Source: CAD feature listing. Evaluate the final solid. Frame: model axes, mm. A direction names the side the tool comes from. Give positions to 0.01 mm unless a question says otherwise; leave off trailing zeros. Order: outer loops, then holes, each group sorted by start corner. A loop starts at its lowest first (then second) coordinate and runs counter-clockwise, first axis right, second up.
Autodesk Inventor part; units mm, degrees
ref_plane "bolt4_1_XY" through (-10, 3.5, 10) normal (0, 1, 0) x (1, 0, 0)
ref_plane "bolt4_1_YZ" through (-10, 3.5, 10) normal (1, 0, 0) x (0, 0, -1)
ref_plane "bolt4_1_ZX" through (-10, 3.5, 10) normal (0, 0, -1) x (0, 1, 0)
sketch "Sketch_4" plane through (0, 0, 0) normal (0, 1, 0) x (-1, 0, 0)
  line L0 (40, -19) -> (40, 19)
  line L1 (40, 19) -> (39, 20)
  line L2 (39, 20) -> (-39, 20)
  line L3 (-39, 20) -> (-40, 19)
  line L4 (-40, 19) -> (-40, -19)
  line L5 (-40, -19) -> (-39, -20)
  line L6 (-39, -20) -> (39, -20)
  line L7 (39, -20) -> (40, -19)
extrude "Extrusion1" add sketch "Sketch_4" along normal blind 9
sketch "Sketch2" plane through (0, 0, 0) normal (0, -1, 0) x (1, 0, 0)
  point P0 (-30, 10)
hole "Hole1" at (-30, 0, 10) direction (0, 1, 0) diameter 5.5 depth 9 counterbore diameter 9.5 counterbore depth 5.5
pattern_linear "Rectangular Pattern1" count 2 spacing 60 along (1, 0, 0) count 2 spacing 20 along (0, 0, -1) of "Hole1"
sketch "Sketch3" plane through (0, 9, 0) normal (0, 1, 0) x (1, 0, 0)
  point P0 (-10, -10)
hole "Hole2" at (-10, 9, 10) direction (0, -1, 0) diameter 5.5 depth 9 counterbore diameter 9.5 counterbore depth 5.5
pattern_linear "Rectangular Pattern2" count 2 spacing 20 along (1, 0, 0) count 2 spacing 20 along (0, 0, -1) of "Hole2"
ref_plane "bolt4_1_XY" through (-10, 3.5, 10) normal (0, 1, 0) x (1, 0, 0)
ref_plane "bolt4_1_YZ" through (-10, 3.5, 10) normal (1, 0, 0) x (0, 0, -1)
ref_plane "bolt4_1_ZX" through (-10, 3.5, 10) normal (0, 0, -1) x (0, 1, 0)
ref_plane "bolt4_2_XY" through (10, 3.5, 10) normal (0, 1, 0) x (1, 0, 0)
ref_plane "bolt4_2_YZ" through (10, 3.5, 10) normal (1, 0, 0) x (0, 0, -1)
ref_plane "bolt4_2_ZX" through (10, 3.5, 10) normal (0, 0, -1) x (0, 1, 0)
ref_plane "bolt4_3_XY" through (-10, 3.5, -10) normal (0, 1, 0) x (1, 0, 0)
ref_plane "bolt4_3_YZ" through (-10, 3.5, -10) normal (1, 0, 0) x (0, 0, -1)
ref_plane "bolt4_3_ZX" through (-10, 3.5, -10) normal (0, 0, -1) x (0, 1, 0)
ref_plane "bolt4_4_XY" through (10, 3.5, -10) normal (0, 1, 0) x (1, 0, 0)
ref_plane "bolt4_4_YZ" through (10, 3.5, -10) normal (1, 0, 0) x (0, 0, -1)
ref_plane "bolt4_4_ZX" through (10, 3.5, -10) normal (0, 0, -1) x (0, 1, 0)
ref_plane "bolt5_1_XY" through (-30, 5.5, 10) normal (0, 1, 0) x (1, 0, 0)
ref_plane "bolt5_1_YZ" through (-30, 5.5, 10) normal (1, 0, 0) x (0, 0, -1)
ref_plane "bolt5_1_ZX" through (-30, 5.5, 10) normal (0, 0, -1) x (0, 1, 0)
ref_plane "bolt5_2_XY" through (30, 5.5, 10) normal (0, 1, 0) x (1, 0, 0)
ref_plane "bolt5_2_YZ" through (30, 5.5, 10) normal (1, 0, 0) x (0, 0, -1)
ref_plane "bolt5_2_ZX" through (30, 5.5, 10) normal (0, 0, -1) x (0, 1, 0)
ref_plane "bolt5_3_XY" through (-30, 5.5, -10) normal (0, 1, 0) x (1, 0, 0)
ref_plane "bolt5_3_YZ" through (-30, 5.5, -10) normal (1, 0, 0) x (0, 0, -1)
ref_plane "bolt5_3_ZX" through (-30, 5.5, -10) normal (0, 0, -1) x (0, 1, 0)
ref_plane "bolt5_4_XY" through (30, 5.5, -10) normal (0, 1, 0) x (1, 0, 0)
ref_plane "bolt5_4_YZ" through (30, 5.5, -10) normal (1, 0, 0) x (0, 0, -1)
ref_plane "bolt5_4_ZX" through (30, 5.5, -10) normal (0, 0, -1) x (0, 1, 0)
ref_plane "bracket_XY" through (0, 9, 0) normal (0, 1, 0) x (1, 0, 0)
ref_plane "bracket_YZ" through (0, 9, 0) normal (1, 0, 0) x (0, 0, -1)
ref_plane "bracket_ZX" through (0, 9, 0) normal (0, 0, -1) x (0, 1, 0)
properties part number "HBLPL5-4040"
1) Draft query along Z for faces 4 (the cylindrical face through (9.17, 1.73, 12.62)), 5 (the flat face through (1, 4, -20)), 6 (the flat face through (10, 3.5, -7)), 7 (the flat face through (1, 0, 0)). Return one class per face: +Z half, -Z half, draft (parallel to the pull), parting line (faces both ways), or undercut.
Report:
face 4: undercut
face 5: -Z half
face 6: undercut
face 7: draft
2) Material intervals for L1, parallel to X at y = 8, z = 10; L2, parallel to Z at x = 10, y = 6.5; L3, parallel to Z at x = 30, y = 6.55, sorted ascending.
Report:
L1: x = -40 to -32.75, -27.25 to -14.75, -5.25 to 5.25, 14.75 to 27.25, 32.75 to 40
L2: z = -20 to -14.75, -5.25 to 5.25, 14.75 to 20
L3: z = -20 to -12.75, -7.25 to 7.25, 12.75 to 20
3) Reachability of faces 1 (the flat face through (13, 3.5, 10)), 2 (the flat face through (-27, 5.5, 10)), 3 (the flat face through (-40, 4, 0)) from +Z, -Z, +X, -X, +Y, -Y: full face, straight path, thin tool, end or side. Return the list, or none.
Report:
face 1: +Y
face 2: -Y
face 3: +Z, -Z, -X, +Y, -Y
4) Section query D-D, the plane x = 6.5. Return the cut outline in (y, z).
Report:
outline: (0, -20) - (9, -20) - (9, -13.21) - (3.5, -13.21) - (3.5, -6.79) - (9, -6.79) - (9, 6.79) - (3.5, 6.79) - (3.5, 13.21) - (9, 13.21) - (9, 20) - (0, 20) - close
5) Section query A-A, the plane x = -30. Return the cut outline in (y, z), and give its area (3 significant figures).
Report:
outline: (0, -20) - (9, -20) - (9, -12.75) - (5.5, -12.75) - (5.5, -14.75) - (0, -14.75) - close; (0, -5.25) - (5.5, -5.25) - (5.5, -7.25) - (9, -7.25) - (9, 7.25) - (5.5, 7.25) - (5.5, 5.25) - (0, 5.25) - close; (0, 14.75) - (5.5, 14.75) - (5.5, 12.75) - (9, 12.75) - (9, 20) - (0, 20) - close
area: 217 mm2
6) Section query B-B, the plane y = 7.75. Count the separate pieces of the cut face and the enclosed holes in it, and give its area (3 significant figures).
Report:
separate pieces: 1
enclosed holes: 8
area: 2,820 mm2
7) Pin query (flat end, axial travel): pin 1 (5 mm diameter, centred on x = -10, z = 10, fed in from -Y); pin 2 (8.5 mm diameter, centred on x = 10, z = -10, fed in from +Y); pin 3 (3 mm diameter, centred on x = -28, z = 8.5, fed in from -Y). Return the tip coordinate at first contact, or that it passes through.
Report:
pin 1: passes through
pin 2: stops at y = 3.5
pin 3: stops at y = 5.5
